Input: part model. Units: mm. Frame: model coordinates. Coordinates: 2 decimals unless noted, no trailing zeros. Order: outer loops, then holes, each group sorted by start corner. A loop starts at its lowest first (then second) coordinate and runs counter-clockwise, first axis right, second up. Notation, with made-up numbers: (12, 82.25) - (49, 82.25) arc R17 ccw to (49, 101.25) - close; hole circle Ø5 at (86.5, -17). An arc over 180 degrees is marked (long way). One line per question, with ' | ' between items.
from build123d import *


with BuildPart() as part:
    # roll_75_sketch → Revolution (revolve)
    with BuildSketch(Plane.XZ):
        Polygon((0, 34.15), (375, 34.15), (375, 10), (455, 10), (455, 0), (0, 0), align=None)
    revolution = revolve(axis=Axis((0, 0, 0), (1, 0, 0)))

    # Mirrored: Revolution across roll_75_sketch V_Axis
    add(revolution.mirror(Plane(origin=(0, 0, 0), x_dir=(0, -1, 0), z_dir=(1, 0, 0))))


solid = part.part
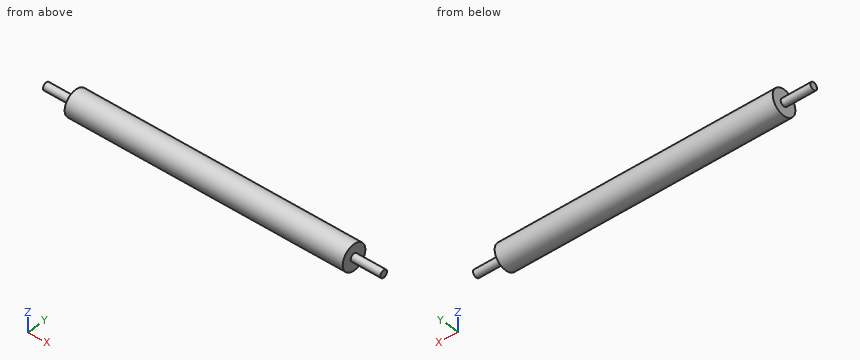
Item 1: Section A-A on y = 0. Return the cut outline in (x, z).
Data:
outline: (-455, -10) - (-375, -10) - (-375, -34.15) - (375, -34.15) - (375, -10) - (455, -10) - (455, 10) - (375, 10) - (375, 34.15) - (-375, 34.15) - (-375, 10) - (-455, 10) - close
Item 2: Contact query for flat-ended pins moving along their axis: P1, Ø6, axis at x = -125, y = 26, coming from the +Z side; P2, Ø4, axis at x = -114.5, y = -20, coming from the -Z side; P3, Ø1.5, axis at x = 298.5, y = 24, coming from the -Z side. Output: stop coordinate, or through.
Data:
P1: z = 25.24 | P2: z = -29.02 | P3: z = -25.01
Item 3: Section C-C on x = -117. Return the cut outline in (y, z), and give its area (3 significant figures).
Data:
outline: circle Ø68.3 at (0, 0) | area: 3,660 mm^2
Item 4: Ray query, line 1 (Z direction, x = -52.5, y = 3.5); line 2 (X direction, y = -22, z = 1.5); line 3 (Z direction, x = -407.5, y = -0.5). Return the intervals inside material, ascending.
Data:
line 1: -33.97 to 33.97 | line 2: -375 to 375 | line 3: -9.99 to 9.99
